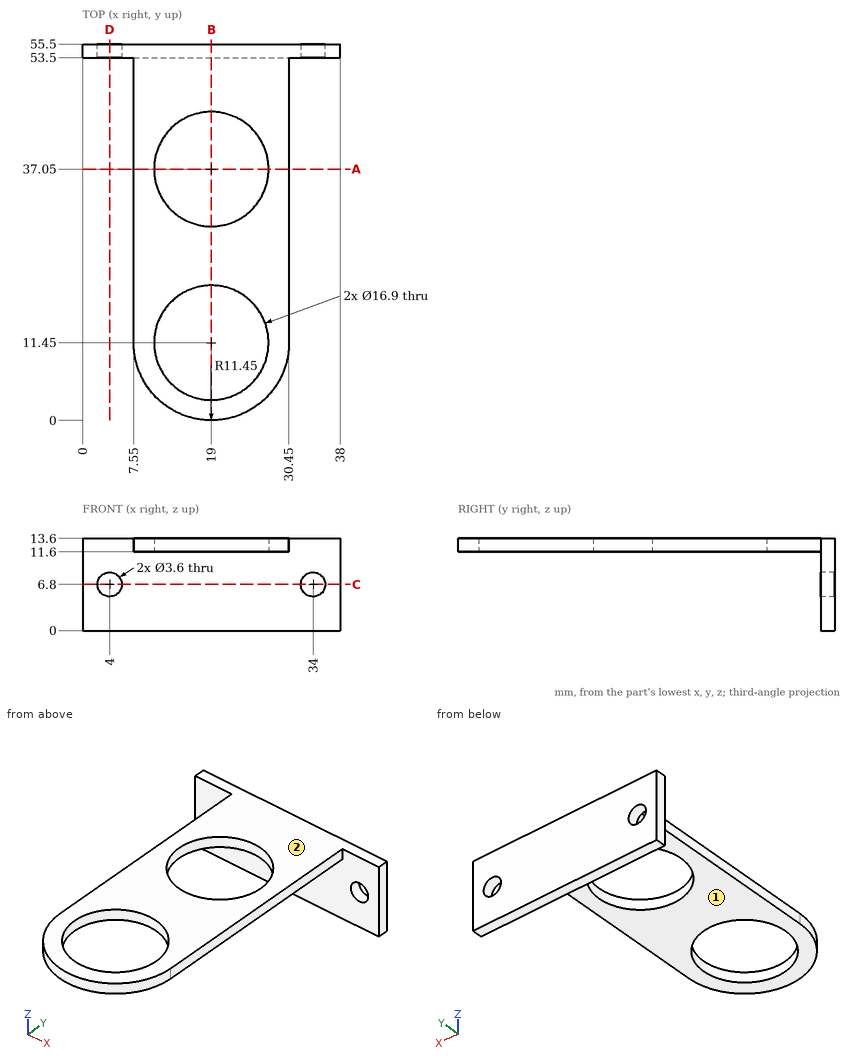
Drawing for the job (mm, zero at the part's lowest x, y, z). A direction names the side the tool comes from. Give positions to 0.01 mm unless a question says otherwise; leave off trailing zeros. Order: outer loops, then holes, each group sorted by start corner. A loop starts at its lowest first (then second) coordinate and runs counter-clockwise, first axis right, second up. Notation, with made-up numbers: (-11, -33) - (19, -33) arc R18 ccw to (19, -23) - close; hole circle Ø4 at (55, 4). An arc over 180 degrees is marked (long way). Write item = value, one per line. Start each with the question number.
1. Cut at A-A, the plane y = 37.05. List the corners of the cut face in (x, z).
2. Which spindle directions (+Z, -Z, +X, -X, +Y, -Y) get a long thin tool onto all of the face, cutting with end or side? Do the marked faces 1 and 2. Say none if no direction does.
3. Drop flat-ended pins along their axis: P1, Ø2, axis at x = 34, z = 6.8, coming from the +Y side; P2, Ø12, axis at x = 20, y = 23, coming from the -Z side; P3, Ø2, axis at y = 30.5, z = 12.5, coming from the +X side; P4, Ø1, axis at y = 32.5, z = 12.5, coming from the -X side. Give the stop position or say it passes through.
4. Cut at D-D, the plane x = 4. List the corners of the cut face in (y, z), and give its area (3 significant figures).
5. Cut at B-B, the plane x = 19. List the corners of the cut face in (y, z), and give its area (3 significant figures).
6. Cut at C-C, the plane z = 6.8. List the corners of the cut face in (x, y).
7. Probe line 1 along Y through (x, z) = (19, 12.5); line 2 along Z through (x, y) = (34, 54.35); line 3 along Y through (x, z) = (28, 7.5). List the from-to ranges inside material, lowest first.
Taken from the geometry:
q1.outline = (7.55, 11.6) - (10.55, 11.6) - (10.55, 13.6) - (7.55, 13.6) - close; (27.45, 11.6) - (30.45, 11.6) - (30.45, 13.6) - (27.45, 13.6) - close
q2.face_1 = -Z, +X, -X, -Y
q2.face_2 = +Z, +X, -X, +Y, -Y
q3.P1 = through
q3.P2 = 11.6
q3.P3 = 30.45
q3.P4 = 7.55
q4.outline = (53.5, 0) - (55.5, 0) - (55.5, 5) - (53.5, 5) - close; (53.5, 8.6) - (55.5, 8.6) - (55.5, 13.6) - (53.5, 13.6) - close
q4.area = 20.0 mm²
q5.outline = (0, 11.6) - (3, 11.6) - (3, 13.6) - (0, 13.6) - close; (19.9, 11.6) - (28.6, 11.6) - (28.6, 13.6) - (19.9, 13.6) - close; (45.5, 11.6) - (53.5, 11.6) - (53.5, 0) - (55.5, 0) - (55.5, 13.6) - (45.5, 13.6) - close
q5.area = 66.6 mm²
q6.outline = (0, 53.5) - (2.2, 53.5) - (2.2, 55.5) - (0, 55.5) - close; (5.8, 53.5) - (32.2, 53.5) - (32.2, 55.5) - (5.8, 55.5) - close; (35.8, 53.5) - (38, 53.5) - (38, 55.5) - (35.8, 55.5) - close
q7.line_1 = 0 to 3, 19.9 to 28.6, 45.5 to 55.5
q7.line_2 = 0 to 5, 8.6 to 13.6
q7.line_3 = 53.5 to 55.5
